Design review of the part shown in the three views and the two pictorial views. Dimensions are in mm from the part's minimum x, y and z. A direction names the side the tool comes from. Coordinates: 2 decimals unless noted, no trailing zeros. Write each loop counter-clockwise with the first axis right and the second up, starting at its lowest first coordinate (ties: lowest second). Pieces come first, ordered by that corner, then holes. Notation, with made-up numbers: (-33.5, 85.5) - (-24.5, 85.5) arc R33 cw to (-24.5, 118.5) - close; hole circle Ø8 at (87.5, 26.5). An arc over 180 degrees is marked (long way). Write each question's results on one line, items separated by ' | '.
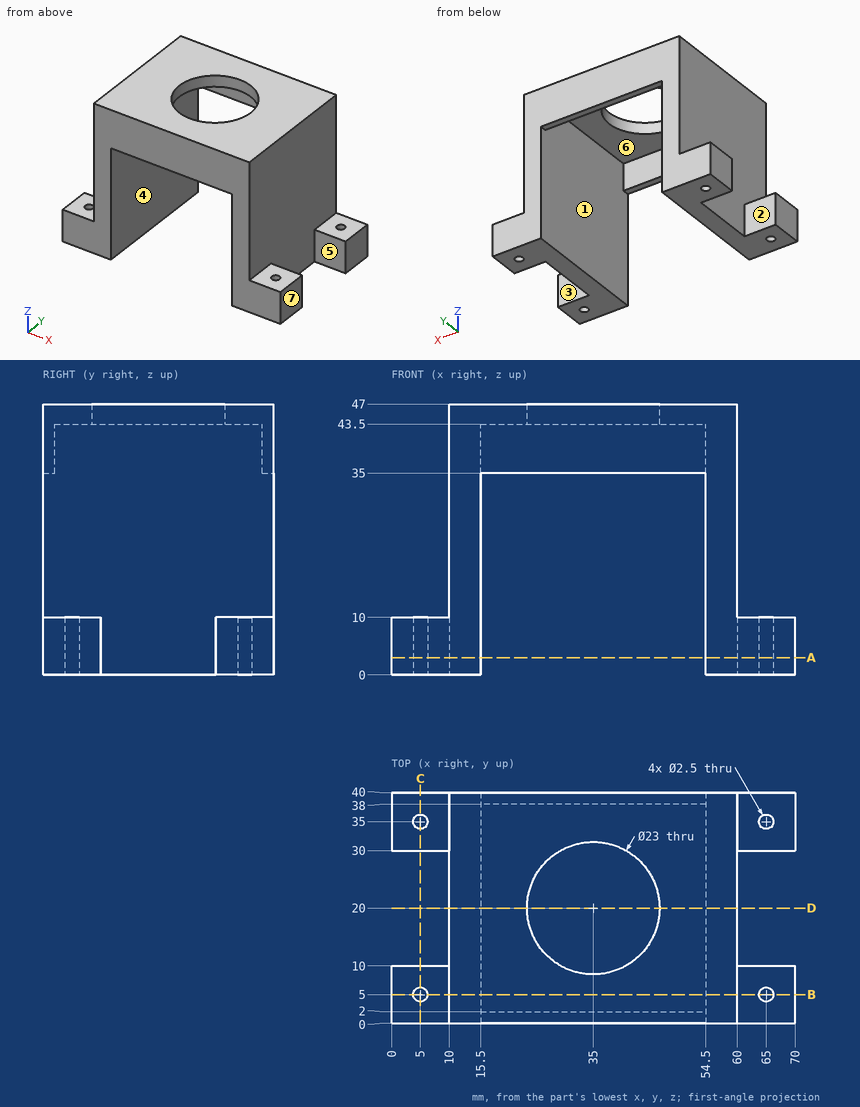
Q1. For pin 1 (12 mm diameter, centred on y = 14.5, z = 34.5, fed in from +X); pin 2 (3 mm diameter, centred on x = 5, y = 35, fed in from +Z); pin 3 (1.5 mm diameter, centred on x = 16.5, z = 10, fed in from +Y); pin 4 (1 mm diameter, centred on y = 27, z = 25.5, fed in from -X), all flat-tipped, find the tip position at first contact; note any pin that passes through.
Results found:
pin 1: x = 60 | pin 2: z = 10 | pin 3: through | pin 4: x = 10
Q2. Take a section at C-C on x = 5. State the section outline as (y, z) points, plus the area to 3 significant figures.
Results found:
outline: (0, 0) - (3.75, 0) - (3.75, 10) - (0, 10) - close; (6.25, 0) - (10, 0) - (10, 10) - (6.25, 10) - close; (30, 0) - (33.75, 0) - (33.75, 10) - (30, 10) - close; (36.25, 0) - (40, 0) - (40, 10) - (36.25, 10) - close | area: 150 mm2
Q3. Take a section at A-A on z = 3. State the section outline as (x, y) points, plus the area to 3 significant figures.
Results found:
outline: (0, 0) - (15.5, 0) - (15.5, 40) - (0, 40) - (0, 30) - (10, 30) - (10, 10) - (0, 10) - close; (54.5, 0) - (70, 0) - (70, 10) - (60, 10) - (60, 30) - (70, 30) - (70, 40) - (54.5, 40) - close; hole circle Ø2.5 at (5, 5); hole circle Ø2.5 at (5, 35); hole circle Ø2.5 at (65, 5); hole circle Ø2.5 at (65, 35) | area: 820 mm2
Q4. For the marked faces 1, 2 and 3, list the 3-axis set-ups (+Z, -Z, +X, -X, +Y, -Y) from which the entire face can be reached by the end or side of a thin tool; tool diameter is ignored.
Results found:
face 1: -Z | face 2: +Z, -Z, -X | face 3: +Z, -Z, +X
Q5. Wall thickness on line 1 along Y through (x, z) = (5, 8); line 2 along X through (y, z) = (26.5, 18); line 3 along Y through (x, z) = (9, 6.5): over which ranges is each line inside the solid? List them lowest first. Write a range as from..to.
Results found:
line 1: 0..3.75, 6.25..10, 30..33.75, 36.25..40 | line 2: 10..15.5, 54.5..60 | line 3: 0..10, 30..40
Q6. Take a section at B-B on y = 5. State the section outline as (x, z) points.
Results found:
outline: (0, 0) - (3.75, 0) - (3.75, 10) - (0, 10) - close; (6.25, 0) - (15.5, 0) - (15.5, 43.5) - (54.5, 43.5) - (54.5, 0) - (63.75, 0) - (63.75, 10) - (60, 10) - (60, 47) - (10, 47) - (10, 10) - (6.25, 10) - close; (66.25, 0) - (70, 0) - (70, 10) - (66.25, 10) - close
Q7. Take a section at D-D on y = 20. State the section outline as (x, z) points.
Results found:
outline: (10, 0) - (15.5, 0) - (15.5, 43.5) - (23.5, 43.5) - (23.5, 47) - (10, 47) - close; (46.5, 43.5) - (54.5, 43.5) - (54.5, 0) - (60, 0) - (60, 47) - (46.5, 47) - close
Q8. Mouldability with a two-part tool opening along X and no side actions: class the marked faces 4, 5, 6 and 7 as pulls with the +X half, pulls with the -X half, needs draft (parallel to the pull), parting line crosses it, or undercut.
Results found:
face 4: undercut | face 5: needs draft | face 6: undercut | face 7: pulls with the +X half
